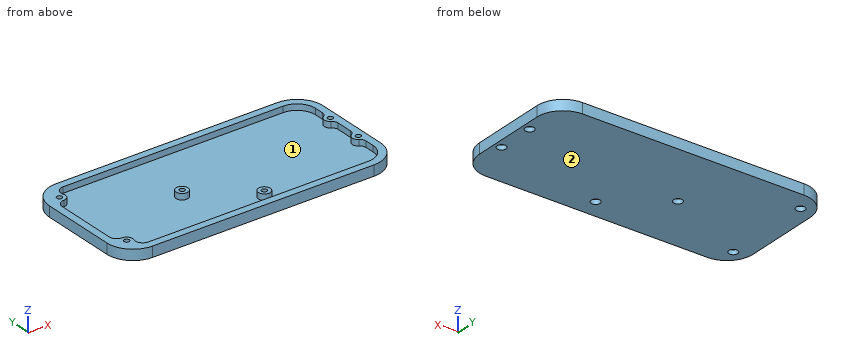
```python
from build123d import *

# Parameters (mm, degrees)
SALIENTE_EXTRUIR1_DEPTH    = 3
CROQUIS2_R                 = 4
SALIENTE_EXTRUIR3_DEPTH    = 4
CORTAR_EXTRUIR1_DEPTH      = 204.311190051
CORTAR_EXTRUIR1_DEPTH_BACK = 204.311190051
CROQUIS3_R                 = 1.75
CROQUIS4_R                 = 3
CORTAR_EXTRUIR2_DEPTH      = 3


with BuildPart() as part:
    # Croquis1 → Saliente-Extruir1 (new body)
    with BuildSketch(Plane.XY):
        with BuildLine():
            Line((17.5, 0), (166.5, 0))
            ThreePointArc((166.5, 0), (178.874368671, 5.125631329), (184, 17.5))
            Line((184, 17.5), (184, 68.7))
            ThreePointArc((184, 68.7), (178.874368671, 81.074368671), (166.5, 86.2))
            Line((166.5, 86.2), (17.5, 86.2))
            ThreePointArc((17.5, 86.2), (5.125631329, 81.074368671), (0, 68.7))
            Line((0, 68.7), (0, 17.5))
            ThreePointArc((0, 17.5), (5.125631329, 5.125631329), (17.5, 0))
        make_face()
    extrude(amount=SALIENTE_EXTRUIR1_DEPTH)

    # Croquis2 → Saliente-Extruir3 (add)
    # profile 1 of 3: a face of its own
    with BuildSketch(Plane.XY.offset(3)):
        with BuildLine():
            ThreePointArc((184, 68.7), (178.874368671, 81.074368671), (166.5, 86.2))
            Line((166.5, 86.2), (17.5, 86.2))
            ThreePointArc((17.5, 86.2), (5.125631329, 81.074368671), (0, 68.7))
            Line((0, 68.7), (0, 17.5))
            ThreePointArc((0, 17.5), (5.125631329, 5.125631329), (17.5, 0))
            Line((17.5, 0), (166.5, 0))
            ThreePointArc((166.5, 0), (178.874368671, 5.125631329), (184, 17.5))
            Line((184, 17.5), (184, 68.7))
        make_face()
        with BuildLine():
            Line((166.5, 5), (18.449260323, 5))
            ThreePointArc((18.449260323, 5), (14.349802364, 7.137405994), (13.75522681, 11.722222222))
            ThreePointArc((13.75522681, 11.722222222), (13.279566367, 15.390075205), (10, 17.1))
            ThreePointArc((10, 17.1), (6.464466094, 18.564466094), (5, 22.1))
            Line((5, 22.1), (5, 64.1))
            ThreePointArc((5, 64.1), (6.464466094, 67.635533906), (10, 69.1))
            ThreePointArc((10, 69.1), (13.279566367, 70.809924795), (13.75522681, 74.477777778))
            ThreePointArc((13.75522681, 74.477777778), (14.349802364, 79.062594006), (18.449260323, 81.2))
            Line((18.449260323, 81.2), (166.5, 81.2))
            ThreePointArc((166.5, 81.2), (175.338834765, 77.538834765), (179, 68.7))
            Line((179, 68.7), (179, 62.52820323))
            ThreePointArc((179, 62.52820323), (178.464101615, 60.52820323), (177, 59.064101615))
            ThreePointArc((177, 59.064101615), (175, 55.6), (177, 52.135898385))
            ThreePointArc((177, 52.135898385), (178.464101615, 50.67179677), (179, 48.67179677))
            Line((179, 48.67179677), (179, 37.52820323))
            ThreePointArc((179, 37.52820323), (178.464101615, 35.52820323), (177, 34.064101615))
            ThreePointArc((177, 34.064101615), (175, 30.6), (177, 27.135898385))
            ThreePointArc((177, 27.135898385), (178.464101615, 25.67179677), (179, 23.67179677))
            Line((179, 23.67179677), (179, 17.5))
            ThreePointArc((179, 17.5), (175.338834765, 8.661165235), (166.5, 5))
        make_face(mode=Mode.SUBTRACT)
    # profile 2 of 3: a face of its own
    with BuildSketch(Plane.XY.offset(3)):
        with Locations(Location((102.5, 13, 0), (0, 0, 180))):
            Circle(CROQUIS2_R)
    # profile 3 of 3: a face of its own
    with BuildSketch(Plane.XY.offset(3)):
        with Locations(Location((67.5, 40, 0), (0, 0, 180))):
            Circle(CROQUIS2_R)
    extrude(amount=SALIENTE_EXTRUIR3_DEPTH)

    # Croquis3 → Cortar-Extruir1 (cut, two sides: drawn at the far end of the back side and taken through both)
    with BuildSketch(Plane.XY.offset(7).offset(-CORTAR_EXTRUIR1_DEPTH_BACK)):
        with Locations((10, 13.1)):
            Circle(CROQUIS3_R)
        with Locations((67.5, 40)):
            Circle(CROQUIS3_R)
        with Locations((102.5, 13)):
            Circle(CROQUIS3_R)
        with Locations((10, 73.1)):
            Circle(CROQUIS3_R)
        with Locations((179, 55.6)):
            Circle(CROQUIS3_R)
        with Locations((179, 30.6)):
            Circle(CROQUIS3_R)
    extrude(amount=CORTAR_EXTRUIR1_DEPTH + CORTAR_EXTRUIR1_DEPTH_BACK, mode=Mode.SUBTRACT)

    # Croquis4 → Cortar-Extruir2 (cut)
    with BuildSketch(Plane(origin=(0, 0, 0), x_dir=(-1, 0, 0), z_dir=(0, 0, -1))):
        with Locations((-179, 30.6)):
            Circle(CROQUIS4_R)
        with Locations((-179, 55.6)):
            Circle(CROQUIS4_R)
        with Locations((-102.5, 13)):
            Circle(CROQUIS4_R)
        with Locations((-67.5, 40)):
            Circle(CROQUIS4_R)
        with Locations((-10, 73.1)):
            Circle(CROQUIS4_R)
        with Locations((-10, 13.1)):
            Circle(CROQUIS4_R)
    extrude(amount=-CORTAR_EXTRUIR2_DEPTH, mode=Mode.SUBTRACT)


solid = part.part
```
Could you check a few things on this model? Use its own coordinates, in mm. Face numbers are marked on the shaded views. Coordinates: 2 decimals unless noted, no trailing zeros. Order: outer loops, then holes, each group sorted by start corner. A loop starts at its lowest first (then second) coordinate and runs counter-clockwise, first axis right, second up. Notation, with made-up numbers: M 78.25,85.25 L 102.25,85.25 A13 cw 102.25,105.25 Z; hole C 14,-39.5 d4. An arc over 180 degrees is marked long. Use a Markdown table: item, result. Add a question column.
Q1. I'm going to push flat-ended pins straight in: pin 1 (2 mm diameter, centred on y = 70.5, z = 3, fed in from -X); pin 2 (4.5 mm diameter, centred on x = 10, y = 73.1, fed in from -Z); pin 3 (3 mm diameter, centred on x = 102.5, y = 13, fed in from +Z); pin 4 (2 mm diameter, centred on x = 157.5, y = 75.5, fed in from +Z). Where does each tip first touch, or does it pass through?
Q2. I want a section at B-B on x = 67.5. List the corners of the cut face in (y, z) for me.
Q3. We'd pull the mould along X, two halves only. Please class the marked faces 1 and 2: pulls with the +X half, pulls with the -X half, needs draft (parallel to the pull), parting line crosses it, or undercut.
Q4. I want a section at D-D on x = 126.5. List the corners of the cut face in (y, z) for me, then the cut area to 3 significant figures.
Q5. If I drill on L1, parallel to Y at x = 67.5, z = 4.45; L2, parallel to Y at x = 102.5, z = 3.9; L3, parallel to X at y = 55.6, z = 5.15, over which ranges is the centre line in solid material (lowest first)?
Q6. I want a section at A-A on y = 55.6. List the corners of the cut face in (x, z) for me.
Q7. I want a section at C-C on z = 1.25. List the corners of the cut face in (x, y) for me.
Checked values:
| question | item | result |
|---|---|---|
| 1 | pin 1 | x = 0.02 |
| 1 | pin 2 | z = 3 |
| 1 | pin 3 | through |
| 1 | pin 4 | z = 3 |
| 2 | outline | M 0,0 L 37,0 L 37,3 L 38.25,3 L 38.25,7 L 36,7 L 36,3 L 5,3 L 5,7 L 0,7 Z; M 41.75,3 L 43,3 L 43,0 L 86.2,0 L 86.2,7 L 81.2,7 L 81.2,3 L 44,3 L 44,7 L 41.75,7 Z |
| 3 | face 1 | undercut |
| 3 | face 2 | needs draft |
| 4 | outline | M 0,0 L 86.2,0 L 86.2,7 L 81.2,7 L 81.2,3 L 5,3 L 5,7 L 0,7 Z |
| 4 | area | 299 mm² |
| 5 | L1 | 0 to 5, 36 to 38.25, 41.75 to 44, 81.2 to 86.2 |
| 5 | L2 | 0 to 5, 9 to 11.25, 14.75 to 17, 81.2 to 86.2 |
| 5 | L3 | 0 to 5, 175 to 177.25, 180.75 to 184 |
| 6 | outline | M 0,0 L 176,0 L 176,3 L 177.25,3 L 177.25,7 L 175,7 L 175,3 L 5,3 L 5,7 L 0,7 Z; M 180.75,3 L 182,3 L 182,0 L 184,0 L 184,7 L 180.75,7 Z |
| 7 | outline | M 0,17.5 A17.5 ccw 17.5,0 L 166.5,0 A17.5 ccw 184,17.5 L 184,68.7 A17.5 ccw 166.5,86.2 L 17.5,86.2 A17.5 ccw 0,68.7 Z; hole C 10,13.1 d6; hole C 10,73.1 d6; hole C 67.5,40 d6; hole C 102.5,13 d6; hole C 179,30.6 d6; hole C 179,55.6 d6 |
